Part model, mm, in its own coordinate system. Face numbers are marked on the shaded views. Round coordinates to 2 decimals unless told otherwise and drop trailing zeros. Loops run counter-clockwise (first coordinate to the right, second up) from the corner with the lowest first, then second, coordinate; pieces in that order, holes last.
(1) Cut at C-C on y = 0. List the corners of the cut face in (x, z), then the cut area to 3 significant figures.
(2) Cut at A-A on y = 27. List the corners of the cut face in (x, z), then the cut area to 3 significant figures.
(3) Cut at D-D on x = 0. List the corners of the cut face in (y, z), then the cut area to 3 significant figures.
(4) Probe probe 1 along Y at (x, z) = (0, 1.3); probe 2 along Y at (x, z) = (15, 0.4); probe 3 along Y at (x, z) = (14, 0.7). List the from-to ranges inside material, lowest first.
(5) Cut at B-B on z = 0.4. List the corners of the cut face in (x, y), then the cut area to 3 significant figures.
(6) Mould opens along Y. For the marked faces 1 and 2 say: +Y half, -Y half, draft (parallel to the pull), parting line (faces both ways), or undercut.
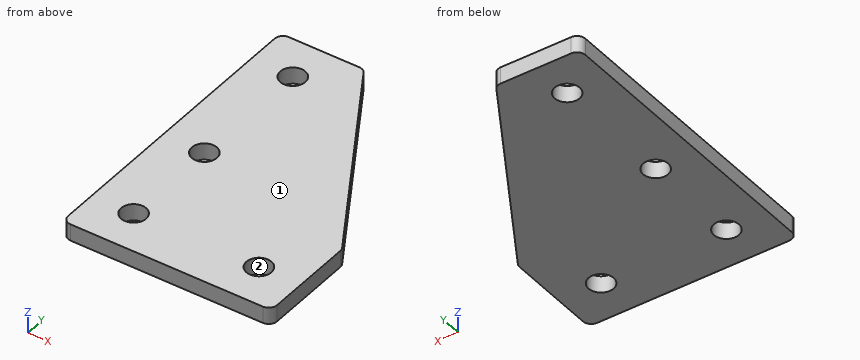
from build123d import *

# Parameters (mm, degrees)
SKETCH_1_R      = 1.5
EXTRUDE_1_DEPTH = 2
FILLET_1_R      = 1


with BuildPart() as part:
    # 草图1 → 凸台-拉伸1 (new body)
    with BuildSketch(Plane.XY):
        Polygon((-5, 32), (5, 32), (20, 7), (20, -5), (-5, -5), align=None)
        with Locations((0, 27)):
            Circle(SKETCH_1_R, mode=Mode.SUBTRACT)
        with Locations((0, 12)):
            Circle(SKETCH_1_R, mode=Mode.SUBTRACT)
        with Locations((15, 0)):
            Circle(SKETCH_1_R, mode=Mode.SUBTRACT)
        Circle(SKETCH_1_R, mode=Mode.SUBTRACT)
    extrude(amount=EXTRUDE_1_DEPTH)

    # 圆角1
    fillet_1_edges = [part.edges().sort_by_distance(p)[0] for p in [
        (-5, 32, 1),
        (5, 32, 1),
        (20, 7, 1),
        (20, -5, 1),
        (-5, -5, 1),
    ]]
    fillet(fillet_1_edges, radius=FILLET_1_R)


solid = part.part
Final values:
1. outline: (-5, 0) - (-1.5, 0) - (-1.5, 2) - (-5, 2) - close; (1.5, 0) - (13.5, 0) - (13.5, 2) - (1.5, 2) - close; (16.5, 0) - (20, 0) - (20, 2) - (16.5, 2) - close
1. area: 38.0 mm2
2. outline: (-5, 0) - (-1.5, 0) - (-1.5, 2) - (-5, 2) - close; (1.5, 0) - (8, 0) - (8, 2) - (1.5, 2) - close
2. area: 20.0 mm2
3. outline: (-5, 0) - (-1.5, 0) - (-1.5, 2) - (-5, 2) - close; (1.5, 0) - (10.5, 0) - (10.5, 2) - (1.5, 2) - close; (13.5, 0) - (25.5, 0) - (25.5, 2) - (13.5, 2) - close; (28.5, 0) - (32, 0) - (32, 2) - (28.5, 2) - close
3. area: 56.0 mm2
4. probe 1: y = -5 to -1.5, 1.5 to 10.5, 13.5 to 25.5, 28.5 to 32
4. probe 2: y = -5 to -1.5, 1.5 to 15.33
4. probe 3: y = -5 to -1.12, 1.12 to 17
5. outline: (-5, -4) arc R1 ccw to (-4, -5) - (19, -5) arc R1 ccw to (20, -4) - (20, 6.72) arc R1 ccw to (19.86, 7.24) - (5.29, 31.51) arc R1 ccw to (4.43, 32) - (-4, 32) arc R1 ccw to (-5, 31) - close; hole circle Ø3 at (0, 0); hole circle Ø3 at (0, 12); hole circle Ø3 at (0, 27); hole circle Ø3 at (15, 0)
5. area: 709 mm2
6. face 1: draft
6. face 2: undercut
